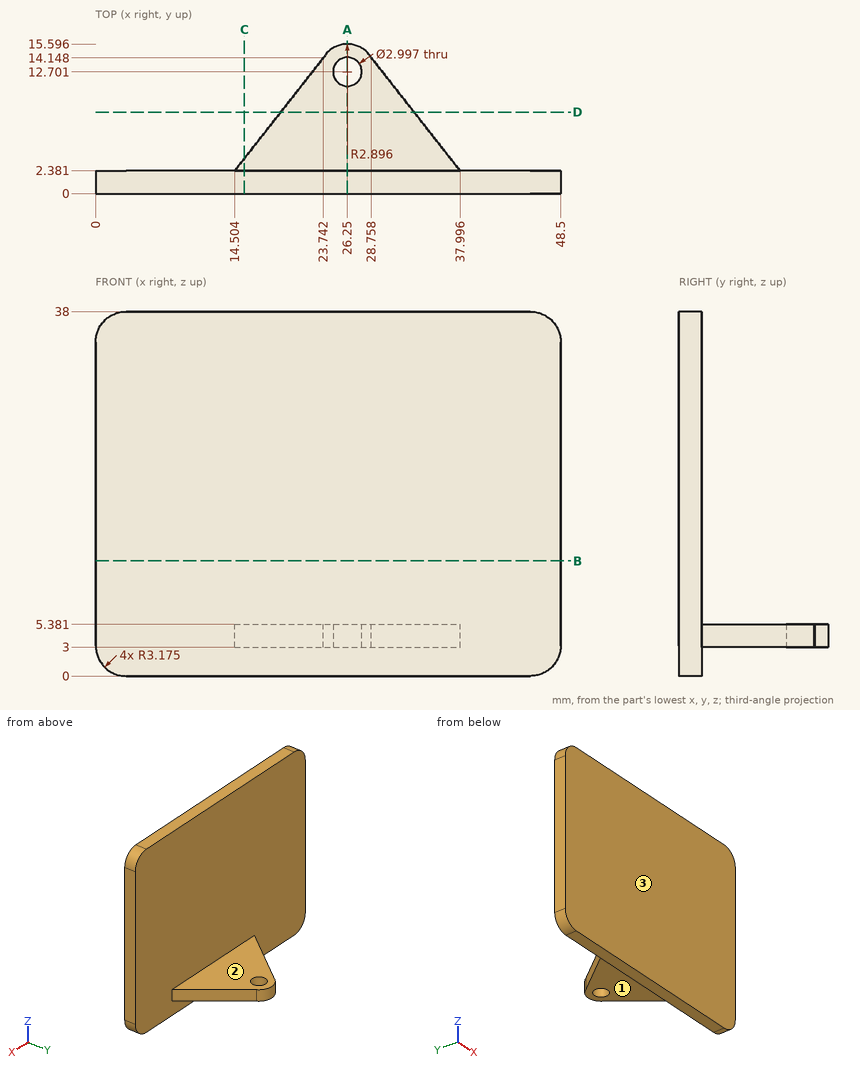
Study the drawing (mm; zero at the part's minimum x, y, z) and answer. A direction names the side the tool comes from. Give positions to 0.01 mm unless a question says otherwise; leave off trailing zeros. Write each loop counter-clockwise with the first axis right and the second up, starting at its lowest first coordinate (ties: lowest second). Pieces come first, ordered by that corner, then holes.
Item 1: Section D-D, the plane y = 8.5 is taken. Write down the section's boundary in (x, z).
Item 2: Section C-C, the plane x = 15.5 is taken. Write down the section's boundary in (y, z).
Item 3: Section A-A, the plane x = 26.25 is taken. Write down the section's boundary in (y, z), plus the area to 3 significant figures.
Item 4: Flat-ended cylindrical pins translate along their axes: P1, Ø3, axis at x = 39, z = 27, coming from the +Y side; P2, Ø4, axis at x = 25, y = 9, coming from the -Z side; P3, Ø4, axis at x = 27.5, y = 6, coming from the +Z side. Find the tip coordinate at first contact, or state that the pin passes through.
Item 5: Find the intervals of material crossed by line 1 along Y through (x, z) = (26.25, 4.25); line 2 along Z through (x, y) = (24, 4.25); line 3 along Y through (x, z) = (25.5, 34.5), in increasing order.
Item 6: Section B-B, the plane z = 12 is taken. Write down the section's boundary in (x, y).
Item 7: Which of the six approach directions +Z, -Z, +X, -X, +Y, -Y give full straight-line access (tool end or side, diameter ignored) to the marked faces 1, 2 and 3?
Completed:
1. outline: (19.31, 3) - (33.19, 3) - (33.19, 5.38) - (19.31, 5.38) - close
2. outline: (0, 0) - (2.38, 0) - (2.38, 3) - (3.65, 3) - (3.65, 5.38) - (2.38, 5.38) - (2.38, 38) - (0, 38) - close
3. outline: (0, 0) - (2.38, 0) - (2.38, 3) - (11.2, 3) - (11.2, 5.38) - (2.38, 5.38) - (2.38, 38) - (0, 38) - close; (14.2, 3) - (15.6, 3) - (15.6, 5.38) - (14.2, 5.38) - close
3. area: 115 mm2
4. P1: stops at y = 2.38
4. P2: stops at z = 3
4. P3: stops at z = 5.38
5. line 1: y = 0 to 11.2, 14.2 to 15.6
5. line 2: z = 3 to 5.38
5. line 3: y = 0 to 2.38
6. outline: (0, 0) - (48.5, 0) - (48.5, 2.38) - (0, 2.38) - close
7. face 1: -Z, +X, -X, +Y
7. face 2: +Z, +X, -X, +Y
7. face 3: +Z, -Z, +X, -X, -Y
